from build123d import *

# Parameters (mm, degrees)
BOSS_EXTRU_1_DEPTH      = 5
ESQUISSE2_W             = 10
ESQUISSE2_H             = 5
ESQUISSE2_W_2           = 5
ESQUISSE2_H_2           = 10
ENL_V_MAT_EXTRU_2_DEPTH = 266.753645318


with BuildPart() as part:
    # Esquisse1 → Boss.-Extru.1 (new body)
    with BuildSketch(Plane.XY):
        Polygon((-250, 10), (150, 10), (150, 90), (250, 90), (250, 10), (250, -10), (-250, -10), align=None)
    extrude(amount=BOSS_EXTRU_1_DEPTH)

    # Esquisse2 → Enlèv. mat.-Extru.2 (cut, through all)
    with BuildSketch(Plane.XY.offset(5)):
        with Locations((-235, 7.5)):
            Rectangle(ESQUISSE2_W, ESQUISSE2_H)
        with Locations((-235, -7.5)):
            Rectangle(ESQUISSE2_W, ESQUISSE2_H)
        with Locations((-215, 7.5)):
            Rectangle(ESQUISSE2_W, ESQUISSE2_H)
        with Locations((-215, -7.5)):
            Rectangle(ESQUISSE2_W, ESQUISSE2_H)
        with Locations((-195, 7.5)):
            Rectangle(ESQUISSE2_W, ESQUISSE2_H)
        with Locations((-195, -7.5)):
            Rectangle(ESQUISSE2_W, ESQUISSE2_H)
        with Locations((-175, 7.5)):
            Rectangle(ESQUISSE2_W, ESQUISSE2_H)
        with Locations((-175, -7.5)):
            Rectangle(ESQUISSE2_W, ESQUISSE2_H)
        with Locations((-155, 7.5)):
            Rectangle(ESQUISSE2_W, ESQUISSE2_H)
        with Locations((-155, -7.5)):
            Rectangle(ESQUISSE2_W, ESQUISSE2_H)
        with Locations((-135, 7.5)):
            Rectangle(ESQUISSE2_W, ESQUISSE2_H)
        with Locations((-135, -7.5)):
            Rectangle(ESQUISSE2_W, ESQUISSE2_H)
        with Locations((-115, 7.5)):
            Rectangle(ESQUISSE2_W, ESQUISSE2_H)
        with Locations((-115, -7.5)):
            Rectangle(ESQUISSE2_W, ESQUISSE2_H)
        with Locations((-95, 7.5)):
            Rectangle(ESQUISSE2_W, ESQUISSE2_H)
        with Locations((-95, -7.5)):
            Rectangle(ESQUISSE2_W, ESQUISSE2_H)
        with Locations((-75, 7.5)):
            Rectangle(ESQUISSE2_W, ESQUISSE2_H)
        with Locations((-75, -7.5)):
            Rectangle(ESQUISSE2_W, ESQUISSE2_H)
        with Locations((-55, 7.5)):
            Rectangle(ESQUISSE2_W, ESQUISSE2_H)
        with Locations((-55, -7.5)):
            Rectangle(ESQUISSE2_W, ESQUISSE2_H)
        with Locations((-35, 7.5)):
            Rectangle(ESQUISSE2_W, ESQUISSE2_H)
        with Locations((-35, -7.5)):
            Rectangle(ESQUISSE2_W, ESQUISSE2_H)
        with Locations((-15, 7.5)):
            Rectangle(ESQUISSE2_W, ESQUISSE2_H)
        with Locations((-15, -7.5)):
            Rectangle(ESQUISSE2_W, ESQUISSE2_H)
        with Locations((5, 7.5)):
            Rectangle(ESQUISSE2_W, ESQUISSE2_H)
        with Locations((5, -7.5)):
            Rectangle(ESQUISSE2_W, ESQUISSE2_H)
        with Locations((25, 7.5)):
            Rectangle(ESQUISSE2_W, ESQUISSE2_H)
        with Locations((25, -7.5)):
            Rectangle(ESQUISSE2_W, ESQUISSE2_H)
        with Locations((45, 7.5)):
            Rectangle(ESQUISSE2_W, ESQUISSE2_H)
        with Locations((45, -7.5)):
            Rectangle(ESQUISSE2_W, ESQUISSE2_H)
        with Locations((65, 7.5)):
            Rectangle(ESQUISSE2_W, ESQUISSE2_H)
        with Locations((65, -7.5)):
            Rectangle(ESQUISSE2_W, ESQUISSE2_H)
        with Locations((85, 7.5)):
            Rectangle(ESQUISSE2_W, ESQUISSE2_H)
        with Locations((85, -7.5)):
            Rectangle(ESQUISSE2_W, ESQUISSE2_H)
        with Locations((105, 7.5)):
            Rectangle(ESQUISSE2_W, ESQUISSE2_H)
        with Locations((105, -7.5)):
            Rectangle(ESQUISSE2_W, ESQUISSE2_H)
        with Locations((125, 7.5)):
            Rectangle(ESQUISSE2_W, ESQUISSE2_H)
        with Locations((125, -7.5)):
            Rectangle(ESQUISSE2_W, ESQUISSE2_H)
        with Locations((145, 7.5)):
            Rectangle(ESQUISSE2_W, ESQUISSE2_H)
        with Locations((145, -7.5)):
            Rectangle(ESQUISSE2_W, ESQUISSE2_H)
        with Locations((165, -7.5)):
            Rectangle(ESQUISSE2_W, ESQUISSE2_H)
        with Locations((185, -7.5)):
            Rectangle(ESQUISSE2_W, ESQUISSE2_H)
        with Locations((205, -7.5)):
            Rectangle(ESQUISSE2_W, ESQUISSE2_H)
        with Locations((225, -7.5)):
            Rectangle(ESQUISSE2_W, ESQUISSE2_H)
        with Locations((247.5, 10)):
            Rectangle(ESQUISSE2_W_2, ESQUISSE2_H_2)
        with Locations((247.5, 30)):
            Rectangle(ESQUISSE2_W_2, ESQUISSE2_H_2)
        with Locations((247.5, 50)):
            Rectangle(ESQUISSE2_W_2, ESQUISSE2_H_2)
        with Locations((247.5, 70)):
            Rectangle(ESQUISSE2_W_2, ESQUISSE2_H_2)
        with Locations((247.5, 90)):
            Rectangle(ESQUISSE2_W_2, ESQUISSE2_H_2)
    extrude(amount=-ENL_V_MAT_EXTRU_2_DEPTH, mode=Mode.SUBTRACT)


solid = part.part
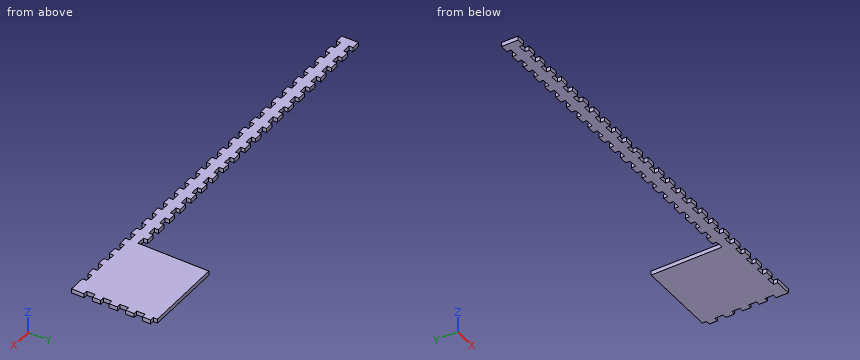
Design review of the part built by this model. Coordinates are the model's own, in mm. Round coordinates to 2 decimals unless told otherwise and drop trailing zeros. Write each loop counter-clockwise with the first axis right and the second up, starting at its lowest first coordinate (ties: lowest second). Pieces come first, ordered by that corner, then holes. Notation, with made-up numbers: (50.5, -9) - (57.5, -9) arc R31 cw to (57.5, 23) - close; hole circle Ø10 at (76.25, 66). An arc over 180 degrees is marked (long way). Use a Markdown table: item, result. Add a question column.
1. Wall thickness on probe 1 along X at (y, z) = (32, 2.1); probe 2 along Y at (x, z) = (54.5, 1.95); probe 3 along X at (y, z) = (43, 4.35): over which ranges is each line inside the solid? List them lowest first.
2. We need section A-A (y = 40). State the section outline as (x, z) points.
3. Clearance check with a flat-ended pin moving along its axis: pin 1 (1.5 mm diameter, centred on x = 26.5, z = 2.5, fed in from -Y). State where the tip first meets the part, or that it passes through.
Output:
| question | item | result |
|---|---|---|
| 1 | probe 1 | x = 150 to 245 |
| 1 | probe 2 | y = -10 to 10 |
| 1 | probe 3 | x = 150 to 250 |
| 2 | outline | (150, 0) - (250, 0) - (250, 5) - (150, 5) - close |
| 3 | pin 1 | stops at y = -5 |
